Input: part model. Units: mm. Frame: model coordinates. Face numbers are marked on the shaded views. A direction names the side the tool comes from. Coordinates: 2 decimals unless noted, no trailing zeros. Loops run counter-clockwise (first coordinate to the right, second up) from the corner with the lowest first, then second, coordinate; pieces in that order, holes last. Notation, with made-up numbers: (88.5, 85.5) -> (147.5, 85.5) arc R16 ccw to (147.5, 92.5) -> close; hole circle Ø10 at (-32.5, 83). An arc over 180 degrees is marked (long way). Answer as a JSON object with one key per item and string values.
from build123d import *

# Parameters (mm, degrees)
ENL_V_MAT_EXTRU_1_DEPTH = 10
BOSS_EXTRU_1_DEPTH      = 8


with BuildPart() as part:
    # Esquisse2 → Base-Révolution (revolve)
    with BuildSketch(Plane(origin=(0, 0, 0), x_dir=(0, 0, -1), z_dir=(1, 0, 0)), mode=Mode.PRIVATE) as base_r_volution_sk:
        Polygon((0, 0), (0, 14), (14, 14), (14, 10), (60, 10), (60, 6), (148, 6), (148, 5), (170, 5), (170, 0), align=None)
    revolve(base_r_volution_sk.sketch.rotate(Axis((0, 0, 67), (0, 0, -1)), 90), axis=Axis((0, 0, 67), (0, 0, -1)))

    # Esquisse3 → Enlèv. mat.-Extru.1 (cut)
    with BuildSketch(Plane.XY):
        Polygon((6.92820323, 0), (3.464101615, 6), (-3.464101615, 6), (-6.92820323, 0), (-3.464101615, -6), (3.464101615, -6), align=None)
    extrude(amount=-ENL_V_MAT_EXTRU_1_DEPTH, mode=Mode.SUBTRACT)

    # Esquisse7 → Boss.-Extru.1 (add)
    with BuildSketch(Plane(origin=(0, 0, -60), x_dir=(-1, 0, 0), z_dir=(0, 0, -1))):
        Polygon((4.838867031, -10.484211901), (11.499027361, -1.051524176), (6.660160329, 9.432687725), (-4.838867031, 10.484211901), (-11.499027361, 1.051524176), (-6.660160329, -9.432687725), align=None)
    extrude(amount=BOSS_EXTRU_1_DEPTH)


solid = part.part
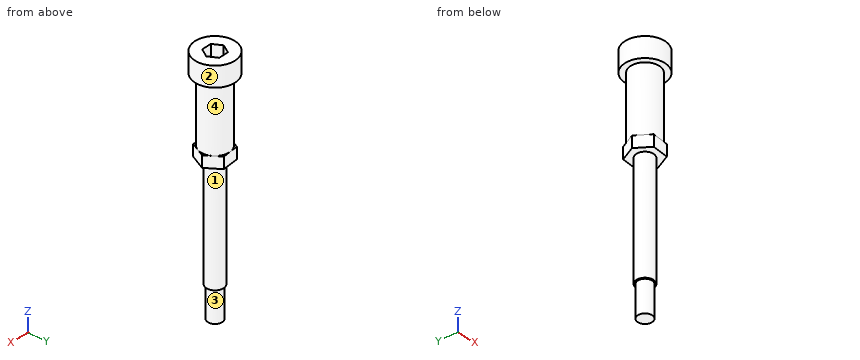
1. Mould query, pull axis Z, two halves, no side actions, for the marked faces 3 and 4. Classes: pulls with the +Z half, pulls with the -Z half, needs draft (parallel to the pull), parting line crosses it, or undercut.
Reply:
{"face 3": "needs draft", "face 4": "undercut"}
2. Access query for the marked faces 1 and 2. Directions: +Z, -Z, +X, -X, +Y, -Y. A direction counts if a zero-diameter tool reaches every point of the face in a straight line with its end or side. Return the directions, or none.
Reply:
{"face 1": "-Z", "face 2": "+Z, -Z"}
3. Line query: line 1 along Z through (x, y) = (2, -4); line 2 along Z through (x, y) = (-2.5, 7); line 3 along Y through (x, z) = (-3.5, -105.5). Output: solid intervals per line, ascending.
Reply:
{"line 1": "z = -170 to -10", "line 2": "z = -68 to 0", "line 3": "y = -4.87 to 4.87"}
4. Section query B-B (z = -37). Return loops of the section in (x, y).
Reply:
{"outline": "circle Ø20 at (0, 0)"}
5. Section query C-C (z = -135). Return loops of the section in (x, y).
Reply:
{"outline": "circle Ø12 at (0, 0)"}
6. Pin query (flat end, axial travel): P1, Ø10, axis at x = 5, y = 0, coming from the +Z side; P2, Ø5, axis at x = 0.5, z = -72.5, coming from the +Y side; P3, Ø1.5, axis at x = 2.5, z = -58, coming from the -Y side; P4, Ø5, axis at x = 4.5, z = -92.5, coming from the -Y side. Return the tip coordinate at first contact, or that it passes through.
Reply:
{"P1": "stops at z = 0", "P2": "stops at y = 6", "P3": "stops at y = -9.85", "P4": "stops at y = -5.66"}
7. Section query A-A (y = 7.5). Return loops of the section in (x, z).
Reply:
{"outline": "(-11.82, -14) -> (-6.61, -14) -> (-6.61, -60) -> (-7.55, -60) -> (-7.55, -68) -> (6.95, -68) -> (6.95, -60) -> (6.61, -60) -> (6.61, -14) -> (11.82, -14) -> (11.82, 0) -> (-11.82, 0) -> close"}
